Check sheet for the modelled part. Datum: model origin and axes. Units: mm. Face numbers are marked on the shaded views. A direction names the side the tool comes from. Coordinates: 2 decimals unless noted, no trailing zeros. Write each loop counter-clockwise with the first axis right and the second up, starting at its lowest first coordinate (ties: lowest second). Pieces come first, ordered by that corner, then holes. Notation, with made-up numbers: (21.5, -2) -> (77.5, -2) arc R3 ccw to (77.5, 3) -> close; hole circle Ø10 at (17, 20). An arc over 180 degrees is marked (long way). One line per item, written item: value. Start each with the question number.
1) Draft check along Z on the marked faces 1, 2 and 3. Enter one of: +Z half, -Z half, draft (parallel to the pull), parting line (faces both ways), or undercut.
2) Sectioned sample at C-C on z = 0. Enter the section's corners in (x, y).
3) Scan lines: line 1 along Z through (x, y) = (-1, 3.4); line 2 along X through (y, z) = (1.6, 0); line 3 along X through (y, z) = (3.5, 1.75). Record each from-to range of solid material in increasing order. Write a range as [from, to].
4) Sectioned sample at B-B on x = 0. Enter the section's corners in (y, z).
5) Sectioned sample at D-D on y = 3.1. Enter the section's corners in (x, z).
6) Set-up check for the marked faces 4 and 5: record each of +Z, -Z, +X, -X, +Y, -Y from which the full face is reachable in a straight line by a thin tool's end or side.
7) Sectioned sample at A-A on y = 1.7. Enter the section's corners in (x, z), plus the area to 3 significant figures.
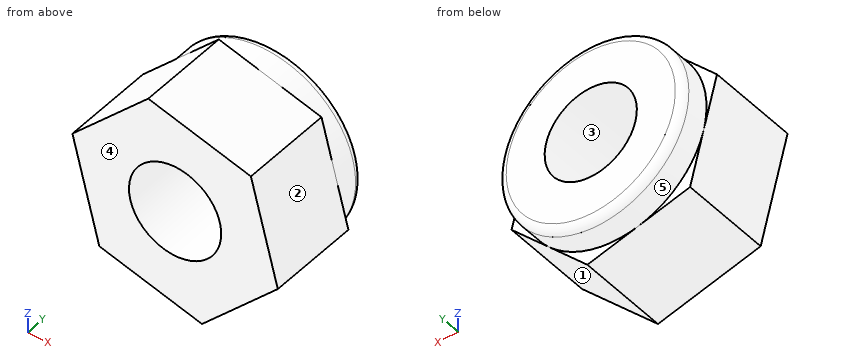
```python
from build123d import *

# Parameters (mm, degrees)
BOSS_EXTRUDE1_DEPTH = 3
SKETCH3_R           = 3
BOSS_EXTRUDE2_DEPTH = 1
CUT_EXTRUDE1_REACH  = 8.196
SKETCH4_R           = 1.5
FILLET1_R           = 0.25


with BuildPart() as part:
    # Sketch1 → Boss-Extrude1 (new body)
    with BuildSketch(Plane(origin=(0, 0, 0), x_dir=(1, 0, 0), z_dir=(0, 1, 0))):
        Polygon((2.465199296, -2.433678786), (3.340227301, 0.918085822), (0.875028005, 3.351764608), (-2.465199296, 2.433678786), (-3.340227301, -0.918085822), (-0.875028005, -3.351764608), align=None)
    extrude(amount=BOSS_EXTRUDE1_DEPTH)

    # Sketch3 → Boss-Extrude2 (add)
    with BuildSketch(Plane(origin=(0, 3, 0), x_dir=(1, 0, 0), z_dir=(0, 1, 0))):
        with Locations(Location((0, 0, 0), (0, 0, 105.368649152))):
            Circle(SKETCH3_R)
    extrude(amount=BOSS_EXTRUDE2_DEPTH)

    # Sketch4 → Cut-Extrude1 (cut, up to next)
    with BuildSketch(Plane(origin=(0, 4, 0), x_dir=(1, 0, 0), z_dir=(0, 1, 0)), mode=Mode.PRIVATE) as cut_extrude1_sk1:
        with Locations(Location((0, 0, 0), (0, 0, 270))):
            Circle(SKETCH4_R)
    cut_extrude1_tool1 = extrude(cut_extrude1_sk1.sketch, amount=-CUT_EXTRUDE1_REACH, mode=Mode.PRIVATE) & part.part
    add(cut_extrude1_tool1.solids().sort_by_distance((0, 4, 0))[0], mode=Mode.SUBTRACT)

    # Fillet1
    fillet1_edges = [part.edges().sort_by_distance(p)[0] for p in [
        (0.795085645, 4, 2.892721697),
    ]]
    fillet(fillet1_edges, radius=FILLET1_R)


solid = part.part
```
Answers:
1. face 1: -Z half
1. face 2: +Z half
1. face 3: undercut
2. outline: (-3.1, 0) -> (-1.5, 0) -> (-1.5, 4) -> (-2.75, 4) arc R0.25 ccw to (-3, 3.75) -> (-3, 3) -> (-3.1, 3) -> close; (1.5, 0) -> (3.1, 0) -> (3.1, 3) -> (3, 3) -> (3, 3.75) arc R0.25 ccw to (2.75, 4) -> (1.5, 4) -> close
3. line 1: z = [-2.83, -1.12], [1.12, 2.83]
3. line 2: x = [-3.1, -1.5], [1.5, 3.1]
3. line 3: x = [-2.44, 2.44]
4. outline: (0, -3.11) -> (3, -3.11) -> (3, -3) -> (3.75, -3) arc R0.25 ccw to (4, -2.75) -> (4, -1.5) -> (0, -1.5) -> close; (0, 1.5) -> (4, 1.5) -> (4, 2.75) arc R0.25 ccw to (3.75, 3) -> (3, 3) -> (3, 3.11) -> (0, 3.11) -> close
5. outline: circle Ø6 at (0, 0); hole circle Ø3 at (0, 0)
6. face 4: +Z, -Z, +X, -X, -Y
6. face 5: +Y
7. outline: (-3.34, 0.92) -> (-2.47, -2.43) -> (0.88, -3.35) -> (3.34, -0.92) -> (2.47, 2.43) -> (-0.88, 3.35) -> close; hole circle Ø3 at (0, 0)
7. area: 24.1 mm2
